from build123d import *

# Parameters (mm, degrees)
SKETCH1_R               = 2.1
BOSS_EXTRUDE1_DEPTH     = 10
SKETCH3_R               = 2.15
CUT_EXTRUDE1_DEPTH      = 10
CUT_EXTRUDE1_DEPTH_BACK = 10
CUT_EXTRUDE2_START      = -6
SKETCH4_R               = 3.75
CUT_EXTRUDE2_DEPTH      = 10
CUT_EXTRUDE3_START      = -2.5
CUT_EXTRUDE3_DEPTH      = 10


with BuildPart() as part:
    # Sketch1 → Boss-Extrude1 (new body)
    with BuildSketch(Plane(origin=(0, 0, 0), x_dir=(1, 0, 0), z_dir=(0, 1, 0))):
        with BuildLine():
            Line((38.355229041, 16.51897107), (22.928326409, 34.904037705))
            ThreePointArc((22.928326409, 34.904037705), (20.891660307, 35.96425897), (18.70183025, 35.273808205))
            Line((18.70183025, 35.273808205), (14.981111589, 32.151754549))
            ThreePointArc((14.981111589, 32.151754549), (14.481497375, 31.928101372), (13.938983386, 32.000996346))
            ThreePointArc((13.938983386, 32.000996346), (-31.802778701, 14.385488935), (-14.829176591, -31.59833139))
            ThreePointArc((-14.829176591, -31.59833139), (-11.579923366, -34.034003552), (-9.567050503, -37.560827652))
            Line((-9.567050503, -37.560827652), (-4.848288245, -52.083684568))
            ThreePointArc((-4.848288245, -52.083684568), (-4.61517148, -52.924262884), (-4.456195885, -53.781958687))
            ThreePointArc((-4.456195885, -53.781958687), (-2.952237368, -56.551823245), (0, -57.655605566))
            ThreePointArc((0, -57.655605566), (2.952237368, -56.551823245), (4.456195885, -53.781958687))
            ThreePointArc((4.456195885, -53.781958687), (4.61517148, -52.924262884), (4.848288245, -52.083684568))
            Line((4.848288245, -52.083684568), (9.567050503, -37.560827652))
            ThreePointArc((9.567050503, -37.560827652), (11.579923366, -34.034003552), (14.829176591, -31.59833139))
            ThreePointArc((14.829176591, -31.59833139), (31.462355963, -15.115527853), (33.935308369, 8.170304209))
            ThreePointArc((33.935308369, 8.170304209), (33.957727399, 8.717234271), (34.264739879, 9.170421255))
            Line((34.264739879, 9.170421255), (37.985458541, 12.292474912))
            ThreePointArc((37.985458541, 12.292474912), (39.045679806, 14.329141013), (38.355229041, 16.51897107))
        make_face()
        with BuildLine():
            Line((-2.5, -53.155605566), (-2.5, -37.155605566))
            ThreePointArc((-2.5, -37.155605566), (-3.630466632, -33.989107261), (-6.510684606, -32.254457226))
            ThreePointArc((-6.510684606, -32.254457226), (0, 32.905), (6.510684606, -32.254457226))
            ThreePointArc((6.510684606, -32.254457226), (3.630466632, -33.989107261), (2.5, -37.155605566))
            Line((2.5, -37.155605566), (2.5, -53.155605566))
            ThreePointArc((2.5, -53.155605566), (0, -55.655605566), (-2.5, -53.155605566))
        make_face(mode=Mode.SUBTRACT)
        with Locations((20.383679412, 30.15801077)):
            Circle(SKETCH1_R, mode=Mode.SUBTRACT)
        with Locations((33.239431606, 14.837121908)):
            Circle(SKETCH1_R, mode=Mode.SUBTRACT)
    extrude(amount=BOSS_EXTRUDE1_DEPTH)

    # Sketch3 → Cut-Extrude1 (cut, two sides)
    with BuildSketch(Plane(origin=(0, 0, 0), x_dir=(0, 0, -1), z_dir=(1, 0, 0))) as cut_extrude1_sk:
        with Locations((-44.82225611, 5)):
            Circle(SKETCH3_R)
    extrude(amount=CUT_EXTRUDE1_DEPTH, mode=Mode.SUBTRACT)
    extrude(cut_extrude1_sk.sketch, amount=-CUT_EXTRUDE1_DEPTH_BACK, mode=Mode.SUBTRACT)

    # Sketch4 → Cut-Extrude2 (cut)
    with BuildSketch(Plane(origin=(0, 0, 0), x_dir=(0, 0, -1), z_dir=(1, 0, 0)).offset(CUT_EXTRUDE2_START)):
        with Locations((-44.82225611, 5)):
            Circle(SKETCH4_R)
    extrude(amount=-CUT_EXTRUDE2_DEPTH, mode=Mode.SUBTRACT)

    # Sketch5 → Cut-Extrude3 (cut)
    with BuildSketch(Plane.ZY.offset(-2.5).offset(CUT_EXTRUDE3_START)):
        Polygon((46.842982052, 8.5), (42.801530168, 8.5), (40.780804226, 5), (42.801530168, 1.5), (46.842982052, 1.5), (48.863707994, 5), align=None)
    extrude(amount=-CUT_EXTRUDE3_DEPTH, mode=Mode.SUBTRACT)


solid = part.part
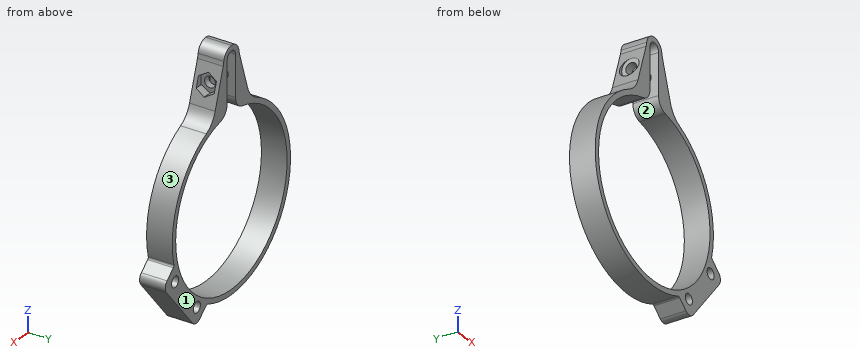
The listing builds one solid part. Answer for the finished solid, in the listing's coordinates (mm). Face numbers are marked on the shaded views. Round coordinates to 2 decimals unless told otherwise and drop trailing zeros. Write each loop counter-clockwise with the first axis right and the second up, starting at its lowest first coordinate (ties: lowest second). Pieces come first, ordered by that corner, then holes. Notation, with made-up numbers: M 61,75.25 L 119,75.25 A25 cw 119,109.25 Z; hole C -18,74 d4. An arc over 180 degrees is marked long. Write each question's results on one line, items separated by ' | '. Start each with the question number.
(1) The part is cut by section B-B, the plane x = -22.5. Write down the section's boundary in (y, z).
(2) Determine the mould class of the marked faces 1, 2 and 3 for opening direction X: +X half, -X half, draft (parallel to the pull), parting line (faces both ways), or undercut.
(3) Find the intervals of material crossed by line 1 (Z direction, x = 4.05, y = 5); line 2 (X direction, y = 3.75, z = -16); line 3 (Z direction, x = 3.9, y = 5), in increasing order.
(4) Each of these flat-tipped pins is pushed along its axis until it touches: P1, Ø6, axis at y = 7, z = 45, coming from the -X side; P2, Ø5, axis at x = 27, y = 1.5, coming from the -Z side; P3, Ø4, axis at y = 7.5, z = 39.5, coming from the +X side; P4, Ø3.5, axis at y = 5, z = 44.82, coming from the -X side. Where does it stop, or does it pass through?
(5) The part is cut by section A-A, the plane z = 0. Write down the section's boundary in (x, y) (3 decimals), and give its area (3 significant figures).
Worked answers:
1) outline: M 0,-26.69 L 10,-26.69 L 10,-24.01 L 0,-24.01 Z; M 0,24.01 L 10,24.01 L 10,26.69 L 0,26.69 Z
2) face 1: draft | face 2: undercut | face 3: +X half
3) line 1: z = -34.67 to -32.65, 33.54 to 42.67, 46.97 to 55.12 | line 2: x = -31.02 to -28.75, 28.75 to 31.49, 34.99 to 38.71 | line 3: z = -34.69 to -32.67, 33.69 to 42.67, 46.97 to 55.4
4) P1: stops at x = -8.11 | P2: stops at z = -33.03 | P3: stops at x = 9.59 | P4: passes through
5) outline: M -34.905,0 L -32.905,0 L -32.905,10 L -34.905,10 Z; M 32.905,0 L 34.905,0 L 34.905,10 L 32.905,10 Z | area: 40.0 mm²
